from build123d import *

# Parameters (mm, degrees)
BOSS_EXTRU_1_DEPTH      = 10
ESQUISSE2_R             = 1
ENL_V_MAT_EXTRU_1_DEPTH = 15


with BuildPart() as part:
    # Esquisse1 → Boss.-Extru.1 (new body)
    with BuildSketch(Plane.XY):
        Polygon((-110.738106784, 134.804121916), (-112.552630047, 133.962988556), (-99.935629642, 106.745139618), (-98.12110638, 107.586272978), (-103.167906542, 118.473412553), (-99.538860017, 120.155679274), (-94.492059855, 109.268539699), (-91.770274961, 110.530239739), (-96.817075123, 121.417379314), (-93.188028598, 123.099646035), (-88.141228436, 112.21250646), (-86.326705174, 113.05363982), (-98.943705578, 140.271488758), (-99.586991765, 136.903720479), (-95.711428679, 128.543215823), (-99.340475204, 126.860949102), (-104.387275366, 137.748088677), (-107.109060259, 136.486388637), (-102.062260098, 125.599249062), (-105.691306623, 123.916982341), align=None)
    extrude(amount=BOSS_EXTRU_1_DEPTH)

    # Esquisse2 → Enlèv. mat.-Extru.1 (cut)
    with BuildSketch(Plane(origin=(-27.920353757, -12.942650812, 0), x_dir=(0, 0, -1), z_dir=(0.9072616312569988, 0.42056668014583565, 0))):
        with Locations(Location((-5, 163.875365486, 0), (0, 0, 90))):
            Circle(ESQUISSE2_R)
        with Locations(Location((-5, 143.875365486, 0), (0, 0, 90))):
            Circle(ESQUISSE2_R)
        with BuildLine():
            Line((0, 138.875365486), (0, 143.875365486))
            ThreePointArc((0, 143.875365486), (-1.464466094, 140.33983158), (-5, 138.875365486))
            Line((-5, 138.875365486), (0, 138.875365486))
        make_face()
        with BuildLine():
            ThreePointArc((-5, 138.875365486), (-8.535533906, 140.33983158), (-10, 143.875365486))
            Line((-10, 143.875365486), (-10, 138.875365486))
            Line((-10, 138.875365486), (-5, 138.875365486))
        make_face()
        with BuildLine():
            Line((-10, 168.875365486), (-10, 163.875365486))
            ThreePointArc((-10, 163.875365486), (-8.535533906, 167.410899392), (-5, 168.875365486))
            Line((-5, 168.875365486), (-10, 168.875365486))
        make_face()
        with BuildLine():
            Line((0, 168.875365486), (-5, 168.875365486))
            ThreePointArc((-5, 168.875365486), (-1.464466094, 167.410899392), (0, 163.875365486))
            Line((0, 163.875365486), (0, 168.875365486))
        make_face()
    extrude(amount=-ENL_V_MAT_EXTRU_1_DEPTH, mode=Mode.SUBTRACT)


solid = part.part
Geometry check sheet. Reference: the model listing, model coordinates, mm. A direction names the side the tool comes from. Give positions to 0.01 mm unless a question says otherwise; leave off trailing zeros. Loops run counter-clockwise (first coordinate to the right, second up) from the corner with the lowest first, then second, coordinate; pieces in that order, holes last.
(1) Section check B-B on y = 122. Record the cut outline in (x, z).
From the geometry:
outline: (-107.01, 0) - (-95.56, 0) - (-95.56, 10) - (-107.01, 10) - close; (-92.68, 0) - (-90.47, 0) - (-90.47, 10) - (-92.68, 10) - close
(2) Section check A-A on y = 128. Record the cut outline in (x, z).
From the geometry:
outline: (-109.79, 0) - (-107.58, 0) - (-107.58, 10) - (-109.79, 10) - close; (-103.18, 0) - (-99.87, 0) - (-99.87, 10) - (-103.18, 10) - close; (-96.88, 0) - (-93.26, 0) - (-93.26, 10) - (-96.88, 10) - close
(3) Release check for a two-part mould opening along Y. For faces 1 (the flat face through (-106.33, 120.54, 4.93)), 2 (the flat face through (-100, 124, 0)), 3 (the flat face through (-101.379, 119.303, 4.93)) record: released by +Y, released by -Y, zero draft, split by the parting line, or undercut.
From the geometry:
face 1: released by -Y
face 2: zero draft
face 3: undercut
(4) Depth check by flat-ended pin: pin 1 Ø2 at (x, z) = (-99, 1.5) entering from -Y; pin 2 Ø5 at (y, z) = (123.5, 5.5) entering from -X; pin 3 Ø3 at (y, z) = (118.5, 8) entering from +X. Enter the tip coordinate at first touch or a pass-through.
From the geometry:
pin 1: stops at y = 107.77
pin 2: stops at x = -108.86
pin 3: stops at x = -88.16
(5) Set-up check for faces 4 (the flat face through (-97.501, 127.714, 4.93)), 5 (the cylindrical face through (-89.73, 118.04, 5.3)), 6 (the flat face through (-99.33, 138.24, 4.94)): record each of +Z, -Z, +X, -X, +Y, -Y from which the full face is reachable in a straight line by a thin tool's end or side.
From the geometry:
face 4: +Z, -Z
face 5: none
face 6: +Z, -Z, +Y
(6) Thickness scan on L1, parallel to Y at x = -102.75, z = 5.5; L2, parallel to X at y = 132, z = 8.75; L3, parallel to Y at x = -96.75, z = 0.5. Record the ranges inside material, lowest first.
From the geometry:
L1: y = 112.82 to 117.57, 118.67 to 125.28, 127.08 to 132.04, 133.95 to 134.22
L2: x = -111.64 to -109.44, -105.03 to -101.72, -97.31 to -95.11
L3: y = 114.14 to 121.27, 121.45 to 128.06, 130.78 to 135.54
(7) Section check D-D on x = -107.75. Record the cut outline in (y, z), then the cut area to 3 significant figures.
From the geometry:
outline: (123.6, 0) - (128.36, 0) - (128.36, 10) - (123.6, 10) - close
area: 47.6 mm2
(8) Section check C-C on z = 7. Record the cut outline in (x, y), then the cut area to 3 significant figures.
From the geometry:
outline: (-112.38, 133.58) - (-100.11, 107.12) - (-98.3, 107.96) - (-103.17, 118.47) - (-99.54, 120.16) - (-94.67, 109.65) - (-91.95, 110.91) - (-96.82, 121.42) - (-93.19, 123.1) - (-88.32, 112.59) - (-86.5, 113.43) - (-98.77, 139.89) - (-99.04, 139.77) - (-99.59, 136.9) - (-95.71, 128.54) - (-99.34, 126.86) - (-104.21, 137.37) - (-106.93, 136.11) - (-102.06, 125.6) - (-105.69, 123.92) - (-110.56, 134.43) - close
area: 250 mm2
